Autodesk Inventor part; units mm, degrees
ref_plane "YZ Plane" through (0, 0, 0) normal (1, 0, 0) x (0, 1, 0)
ref_plane "XZ Plane" through (0, 0, 0) normal (0, 1, 0) x (-1, 0, 0)
ref_plane "XY Plane" through (0, 0, 0) normal (0, 0, 1) x (1, 0, 0)
sketch "スケッチ1" plane through (0, 0, 0) normal (0, 0, 1) x (1, 0, 0)
  line L0 (-297.7333, 0) -> (297.7333, 0) construction
  line L1 (297.7333, 0) -> (297.7333, 0)
  line L2 (227.7333, 70) -> (-227.7333, 70)
  line L3 (-297.7333, 0) -> (-297.7333, 0)
  line L4 (0, 0) -> (0, 70) construction
  line L5 (-227.7333, 70) -> (-297.7333, 0)
  line L6 (227.7333, 70) -> (297.7333, 0)
  line L7 (-297.7333, 0) -> (297.7333, 0) construction
  line L8 (297.7333, 0) -> (297.7333, -40)
  line L9 (293.7333, -67.2) -> (-297.7333, -67.2) construction
  line L10 (-297.7333, -67.2) -> (-297.7333, -40) construction
  line L11 (-297.7333, -40) -> (297.7333, -40)
  line L12 (297.7333, -40) -> (293.7333, -40)
  line L13 (293.7333, -40) -> (293.7333, -67.2)
  line L14 (-297.7333, -40) -> (-297.7333, 0)
  point P0 (297.7333, 70)
  point P1 (-297.7333, 70)
  point P2 (0, 0)
  dimension "d0" = 70
  dimension "d1" = 595.4667
  dimension "d3" = 70
  dimension "d4" = 70
  dimension "d5" = 70
  dimension "d6" = 70
  dimension "d7" = 67.2
  dimension "d10" = 40
  dimension "d12" = 4
extrude "押し出し1" add sketch "スケッチ1" along normal blind 4
properties part number "泥除け2"
Part model, mm, in its own coordinate system. Give positions to 0.01 mm unless a question says otherwise; leave off trailing zeros. Order: outer loops, then holes, each group sorted by start corner. A loop starts at its lowest first (then second) coordinate and runs counter-clockwise, first axis right, second up. Notation, with made-up numbers: (44.25, 63.5) -> (82.25, 63.5) arc R13 ccw to (82.25, 88.5) -> close; hole circle Ø9 at (-18.5, -0.5). An arc over 180 degrees is marked (long way). Use one line per item in the form item = value.
(1) Pull direction Z, two halves, no side cores. Call faces 1 (the face through (-4, 16, 0)), 2 (the face through (-262.243, 35.49, 1.972)), 3 (the face through (-4, 16, 4)): +Z half, -Z half, draft (parallel to the pull), parting line (faces both ways), or undercut.
Solution:
face_1 = -Z half
face_2 = draft
face_3 = +Z half
(2) Saw through at B-B (y = 28). Write the cut outline in (x, z).
Solution:
outline = (-269.73, 0) -> (269.73, 0) -> (269.73, 4) -> (-269.73, 4) -> close
(3) Saw through at A-A (z = 2.8). Write the cut outline in (x, y), then the cut area to 3 significant figures.
Solution:
outline = (-297.73, -40) -> (297.73, -40) -> (297.73, 0) -> (227.73, 70) -> (-227.73, 70) -> (-297.73, 0) -> close
area = 60,600 mm²
(4) Saw through at C-C (y = 51). Write the cut outline in (x, z), then the cut area to 3 significant figures.
Solution:
outline = (-246.73, 0) -> (246.73, 0) -> (246.73, 4) -> (-246.73, 4) -> close
area = 1,970 mm²
(5) Drill centre lines: line 1 (Y direction, x = -269, z = 3.3); line 2 (X direction, y = 57.5, z = 2.45); line 3 (X direction, y = 57, z = 2.8). Where is each one in solid material? Low to high. Write a range as from..to.
Solution:
line_1 = -40..28.73
line_2 = -240.23..240.23
line_3 = -240.73..240.73
